Can you work these out from the model? Positions are in its coordinate system, mm. A direction names the side the tool comes from. Coordinates: 2 decimals unless noted, no trailing zeros. Order: outer loops, then holes, each group sorted by start corner. A loop starts at its lowest first (then second) coordinate and runs counter-clockwise, first axis right, second up. Notation, with made-up numbers: M 2,-18.75 L 54,-18.75 A17 ccw 54,13.25 Z; hole C 11.5,63 d1. An arc over 180 degrees is marked long. Answer as CSV lines item,"result". Start each with the question number.
1. On a 3-axis mill with a long thin cutter (end or side, diameter ignored), from which of +Z, -Z, +X, -X, +Y, -Y can I reach the whole of each face in a straight line? I mean faces 4 (the face through (-32, 206, -3.175)), 5 (the face through (193.542, 125.222, -0.133)). Say none if no direction works.
2. Will these pins go through, and if not, where does the flat tip stop? pin 1 (3 mm diameter, centred on x = -25.5, z = -7, fed in from +Y) (3 decimals); pin 2 (6 mm diameter, centred on y = 198, z = 0.5, fed in from +X) (3 decimals); pin 3 (7 mm diameter, centred on y = 208, z = -6, fed in from +X) (3 decimals).
3. I need wall thicknesses on line 1 along Z through (x, y) = (122.5, 201) (3 decimals); line 2 along Y through (x, z) = (-55.5, 5.5); line 3 along Y through (x, z) = (58, -3.5). Which ranges of each line are inside material? Lowest first, please. Write a range as from..to.
4. If we section it at D-D (z = 2): List the corners of the cut face in (x, y) for me (3 decimals).
5. If we section it at B-B (y = 95.5): List the corners of the cut face in (x, z) for me (3 decimals), plus the area to 3 significant figures.
6. If we mould it in two halves opening along Y, with no side actions, what happens to faces 1 (the face through (-32, 28, -3.175)), 2 (the face through (-3, 0, 0)), 3 (the face through (-2.845, 244.608, 0.133))? For each: released by +Y, released by -Y, zero draft, split by the parting line, or undercut.
```python
from build123d import *

# Parameters (mm, degrees)
F1_DEPTH = 254
F2_SIZE  = 19.04999
F3_W     = 63.5
F3_H     = 19.05
F4_DEPTH = 6.35


# Not quite as in the source:
# - a fillet or chamfer is up to 0.001 mm smaller than in the source, because OpenCascade refuses the exact size


with BuildPart() as f1:
    # F0 (on Front) → F1 (new body)
    with BuildSketch(Plane.XZ):
        Polygon((203.2, 9.525), (-203.2, 9.525), (-184.15, -9.525), (184.15, -9.525), align=None)
    extrude(amount=-F1_DEPTH)

    # F2 (size 19.05 in the source; OpenCascade refuses exactly that, so slightly less here)
    f2_edges = [f1.edges().sort_by_distance(p)[0] for p in [
        (0, 254, -9.525),
    ]]
    chamfer(f2_edges, length=F2_SIZE)

    # F3 (on face) → F4 (cut)
    with BuildSketch(Plane(origin=(0, 0, -9.525), x_dir=(1, 0, 0), z_dir=(0, 0, -1))):
        with Locations((-31.75, -206.375)):
            Rectangle(F3_W, F3_H)
        with Locations((-31.75, -28.575)):
            Rectangle(F3_W, F3_H)
        with Locations((152.4, -28.575)):
            Rectangle(F3_W, F3_H)
        with Locations((152.4, -206.375)):
            Rectangle(F3_W, F3_H)
    extrude(amount=-F4_DEPTH, mode=Mode.SUBTRACT)


solid = f1.part
```
Solved:
1,face 4,"-Z"
1,face 5,"-Z, +X, +Y, -Y"
2,pin 1,"y = 238.975"
2,pin 2,"x = 197.175"
2,pin 3,"x = 191.175"
3,line 1,"-3.175..9.525"
3,line 2,"0..249.98"
3,line 3,"0..240.98"
4,outline,"M -195.675,0 L 195.675,0 L 195.675,246.475 L -195.675,246.475 Z"
5,outline,"M -203.2,9.525 L -184.15,-9.525 L 184.15,-9.525 L 203.2,9.525 Z"
5,area,"7,380 mm²"
6,face 1,"undercut"
6,face 2,"released by -Y"
6,face 3,"released by +Y"
